```python
from build123d import *

# Parameters (mm, degrees)
F1_DEPTH = 2.75
F2_W     = 30
F2_H     = 5
F3_DEPTH = 1.95
F4_SIZE  = 8.24999
F5_SIZE  = 1
F6_R     = 2.74999
F8_D     = 3


# Not quite as in the source:
# - a fillet or chamfer is up to 0.001 mm smaller than in the source, because OpenCascade refuses the exact size


with BuildPart() as f1:
    # F0 (on Top) → F1 (new body, symmetric)
    with BuildSketch(Plane.XY):
        Polygon((-15, 17), (-15, 12), (-15, 4.65), (-6.75, 4.65), (-6.75, -17), (-4.25, -17), (-4.25, -9.2), (-1.25, -9.2), (-1.25, -17), (1.25, -17), (1.25, -9.2), (4.25, -9.2), (4.25, -17), (6.75, -17), (6.75, 4.65), (15, 4.65), (15, 12), (15, 17), align=None)
    extrude(amount=F1_DEPTH, both=True)

    # F2 (on face) → F3 (join)
    with BuildSketch(Plane(origin=(0, 0, -2.75), x_dir=(1, 0, 0), z_dir=(0, 0, -1))):
        with Locations((0, -14.5)):
            Rectangle(F2_W, F2_H)
    extrude(amount=F3_DEPTH)

    # F4 (size 8.25 in the source; OpenCascade refuses exactly that, so slightly less here)
    f4_edges = [f1.edges().sort_by_distance(p)[0] for p in [
        (-15, 4.65, 0),
        (15, 4.65, 0),
    ]]
    chamfer(f4_edges, length=F4_SIZE)

    # F5
    f5_edges = [f1.edges().sort_by_distance(p)[0] for p in [
        (15, 17, -0.975),
        (-15, 17, -0.975),
    ]]
    chamfer(f5_edges, length=F5_SIZE)

    # F6 (radius 2.75 in the source; OpenCascade refuses exactly that, so slightly less here)
    f6_edges = [f1.edges().sort_by_distance(p)[0] for p in [
        (5.5, -17, 2.75),
        (0, -17, 2.75),
        (-5.5, -17, 2.75),
        (5.5, -17, -2.75),
        (0, -17, -2.75),
        (-5.5, -17, -2.75),
    ]]
    fillet(f6_edges, radius=F6_R)

    # F8 (through all)
    with Locations(Plane.YZ.offset(6.75)):
        with Locations((-14.25, 0)):
            Hole(F8_D / 2)


solid = f1.part
```
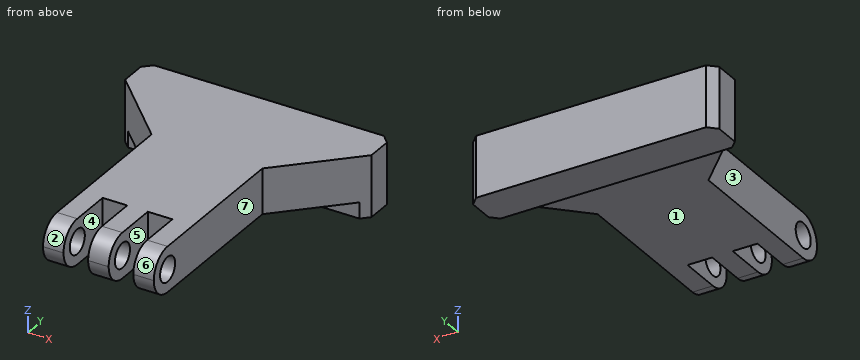
Check sheet for the modelled part. Datum: model origin and axes. Units: mm. Face numbers are marked on the shaded views. A direction names the side the tool comes from. Coordinates: 2 decimals unless noted, no trailing zeros. Order: outer loops, then holes, each group sorted by start corner. A loop starts at its lowest first (then second) coordinate and runs counter-clockwise, first axis right, second up. Notation, with made-up numbers: M -18.5,86.5 L 15.5,86.5 A31 cw 15.5,112.5 Z; hole C -34,46.25 d4. An arc over 180 degrees is marked long. Write each question's results on one line, items separated by ' | '. Start each with the question number.
1. Material ranges on probe 1 along X at (y, z) = (-10.5, -1.25); probe 2 along Z at (x, y) = (-0.2, -14.25); probe 3 along X at (y, z) = (12, -0.5), recorded low to high.
2. Cross-section at A-A on x = -12.75. Record the cut outline in (y, z).
3. Cross-section at D-D on x = 2.75. Record the cut outline in (y, z), and give its area (3 significant figures).
4. Mould release check, pull along X, two halves, no side actions. Record for the marked faces 4, 5, 6 and 7: +X half, -X half, draft (parallel to the pull), parting line (faces both ways), or undercut.
5. Access from +Z, -Z, +X, -X, +Y, -Y to the whole of each face (thin tool, end or side, straight path). Record for the marked faces 1, 2 and 3.
6. Go/stop test with flat-tipped pins: P1, Ø3, axis at y = 11.5, z = 1.5, coming from the +X side; P2, Ø1.6, axis at y = -12, z = 0.5, coming from the +X side; P3, Ø4, axis at x = 6, z = -3, coming from the -Y side; P4, Ø2, axis at x = 6, z = -3.5, coming from the -Y side. Record where each tip stops, or that it passes through.
7. Cross-section at C-C on y = 2. Record the cut outline in (x, z), and give its area (4 significant figures).
Checks:
1) probe 1: x = -6.75 to -4.25, -1.25 to 1.25, 4.25 to 6.75 | probe 2: z = -2.75 to -1.5, 1.5 to 2.75 | probe 3: x = -14.1 to 14.1
2) outline: M 10.65,-2.75 L 12,-2.75 L 12,-4.7 L 17,-4.7 L 17,2.75 L 10.65,2.75 Z
3) outline: M -9.2,-2.75 L 12,-2.75 L 12,-4.7 L 17,-4.7 L 17,2.75 L -9.2,2.75 Z | area: 154 mm²
4) face 4: undercut | face 5: undercut | face 6: draft | face 7: +X half
5) face 1: -Z, +X, -X, -Y | face 2: +Z, +X, -X, -Y | face 3: +Z, -Z, -X, -Y
6) P1: stops at x = 15 | P2: stops at x = 6.75 | P3: stops at y = -16.81 | P4: stops at y = -15.4
7) outline: M -6.75,-2.75 L 6.75,-2.75 L 6.75,2.75 L -6.75,2.75 Z | area: 74.25 mm²
